Read the model definition and answer for the solid it produces. Units are mm, in the model's axes. Coordinates: 2 decimals unless noted, no trailing zeros. Write each loop counter-clockwise with the first axis right and the second up, starting at its lowest first coordinate (ties: lowest second). Pieces come first, ordered by that corner, then holes. Notation, with made-up numbers: (-3.75, 82) -> (44.25, 82) arc R26 cw to (44.25, 98) -> close; hole circle Ø11 at (42.5, 7). An arc over 180 degrees is marked (long way). Answer in a Markdown table with one row per item. Add a question column.
Item 1: Straight lines are drawn through the part: line 1 (X direction, y = 2.25, z = -33); line 2 (X direction, y = -1.75, z = 28); line 3 (X direction, y = -2.25, z = 32.5). For each, find the intervals that lie inside material, in ascending order. Write a range as from..to.
Item 2: Given pin 1 Ø5 at (x, z) = (-57, 30.21) entering from +Y; pin 2 Ø1 at (x, y) = (-25, 0.5) entering from +Z; pin 3 Ø2 at (y, z) = (0, 25) entering from -X, each flat-ended and moving along its own axis, determine where each tip first touches the part or whether it passes through.
Item 3: Section C-C on z = 14 is taken. Write down the section's boundary in (x, y), then the cut area to 3 significant figures.
Item 4: Section D-D on x = -33.5 is taken. Write down the section's boundary in (y, z).
Item 5: Section B-B on x = -43 is taken. Write down the section's boundary in (y, z).
Item 6: Section A-A on y = -1.5 is taken. Count the separate pieces of the cut face and the enclosed holes in it, then the cut area to 3 significant figures.
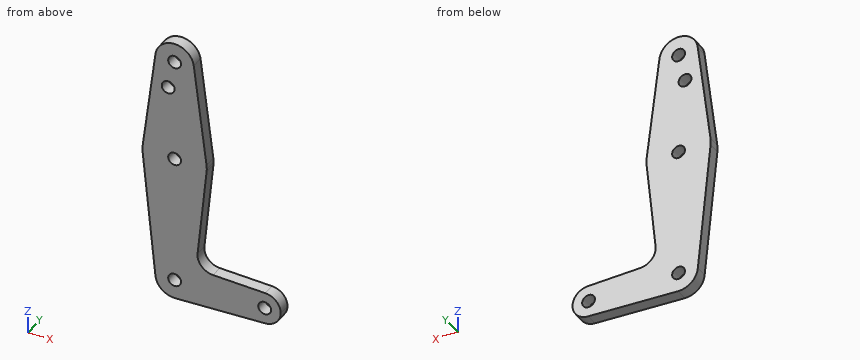
```python
from build123d import *

# Parameters (mm, degrees)
F0_R          = 3.175
F1_DEPTH      = 3.048
F1_DEPTH_BACK = 3.048


with BuildPart() as f1:
    # F0 (on Front) → F1 (new body, two sides)
    with BuildSketch(Plane.XZ) as f1_sk:
        with BuildLine():
            ThreePointArc((-66.490328, 81.796864), (-57.389826, 71.496208), (-47.472626, 81.01313))
            ThreePointArc((-47.472626, 81.01313), (-47.491321, 81.609613), (-47.547333, 82.203755))
            ThreePointArc((-47.547333, 82.203755), (-57.202173, 90.535933), (-66.490328, 81.796864))
        make_face()
        with Locations((-56.997626, 81.01313)):
            Circle(F0_R, mode=Mode.SUBTRACT)
        with BuildLine():
            ThreePointArc((-47.547333, 82.203755), (-47.491321, 81.609613), (-47.472626, 81.01313))
            ThreePointArc((-47.472626, 81.01313), (-57.389826, 71.496208), (-66.490328, 81.796864))
            Line((-66.490328, 81.796864), (-72.747765, 32.200273))
            ThreePointArc((-72.747765, 32.200273), (-56.996231, 46.08813), (-41.247138, 32.197505))
            Line((-41.247138, 32.197505), (-47.547333, 82.203755))
        make_face()
        with Locations((-60.172626, 66.73833)):
            Circle(F0_R, mode=Mode.SUBTRACT)
        with BuildLine():
            ThreePointArc((-41.122626, 30.21313), (-41.153785, 31.207269), (-41.247138, 32.197505))
            ThreePointArc((-41.247138, 32.197505), (-56.996231, 46.08813), (-72.747765, 32.200273))
            ThreePointArc((-72.747765, 32.200273), (-72.871369, 30.412875), (-72.79278, 28.622934))
            ThreePointArc((-72.79278, 28.622934), (-56.996271, 14.33813), (-41.202201, 28.62563))
            ThreePointArc((-41.202201, 28.62563), (-41.142532, 29.418383), (-41.122626, 30.21313))
        make_face()
        with Locations((-56.997626, 30.21313)):
            Circle(F0_R, mode=Mode.SUBTRACT)
        with BuildLine():
            ThreePointArc((-41.202201, 28.62563), (-56.996271, 14.33813), (-72.79278, 28.622934))
            Line((-72.79278, 28.622934), (-66.509378, -33.78907))
            ThreePointArc((-66.509378, -33.78907), (-57.248813, -23.765183), (-47.472626, -33.28687))
            ThreePointArc((-47.472626, -33.28687), (-50.143137, -39.900614), (-56.657215, -42.805785))
            Line((-56.657215, -42.805785), (-12.395022, -41.222903))
            ThreePointArc((-12.395022, -41.222903), (-20.484861, -33.221945), (-12.265221, -25.354396))
            Line((-12.265221, -25.354396), (-38.029298, -24.437165))
            ThreePointArc((-38.029298, -24.437165), (-43.736422, -21.719407), (-45.65679, -15.696978))
            Line((-45.65679, -15.696978), (-41.202201, 28.62563))
        make_face()
        with BuildLine():
            ThreePointArc((-47.472626, -33.28687), (-57.248813, -23.765183), (-66.509378, -33.78907))
            ThreePointArc((-66.509378, -33.78907), (-63.428308, -40.313389), (-56.657215, -42.805785))
            ThreePointArc((-56.657215, -42.805785), (-50.143137, -39.900614), (-47.472626, -33.28687))
        make_face()
        with Locations((-56.997626, -33.28687)):
            Circle(F0_R, mode=Mode.SUBTRACT)
        with BuildLine():
            ThreePointArc((-12.265221, -25.354396), (-20.484861, -33.221945), (-12.395022, -41.222903))
            ThreePointArc((-12.395022, -41.222903), (-6.881269, -38.845315), (-4.610126, -33.28687))
            ThreePointArc((-4.610126, -33.28687), (-6.835993, -27.77496), (-12.265221, -25.354396))
        make_face()
        with Locations((-12.547626, -33.28687)):
            Circle(F0_R, mode=Mode.SUBTRACT)
    extrude(amount=F1_DEPTH)
    extrude(f1_sk.sketch, amount=-F1_DEPTH_BACK)


solid = f1.part
```
Results below:
| question | item | result |
|---|---|---|
| 1 | line 1 | x = -66.59..-60.16, -53.84..-15.71, -9.39..-4.62 |
| 1 | line 2 | x = -72.73..-59.27, -54.72..-41.27 |
| 1 | line 3 | x = -72.71..-59.2, -54.8..-41.29 |
| 2 | pin 1 | passes through |
| 2 | pin 2 | stops at z = -24.88 |
| 2 | pin 3 | stops at x = -72.53 |
| 3 | outline | (-71.32, -3.05) -> (-42.67, -3.05) -> (-42.67, 3.05) -> (-71.32, 3.05) -> close |
| 3 | area | 175 mm2 |
| 4 | outline | (-3.05, -41.98) -> (3.05, -41.98) -> (3.05, -24.6) -> (-3.05, -24.6) -> close |
| 5 | outline | (-3.05, -42.32) -> (3.05, -42.32) -> (3.05, -22.46) -> (-3.05, -22.46) -> close; (-3.05, 10.74) -> (3.05, 10.74) -> (3.05, 46.11) -> (-3.05, 46.11) -> close |
| 6 | separate pieces | 1 |
| 6 | enclosed holes | 5 |
| 6 | area | 3,770 mm2 |
